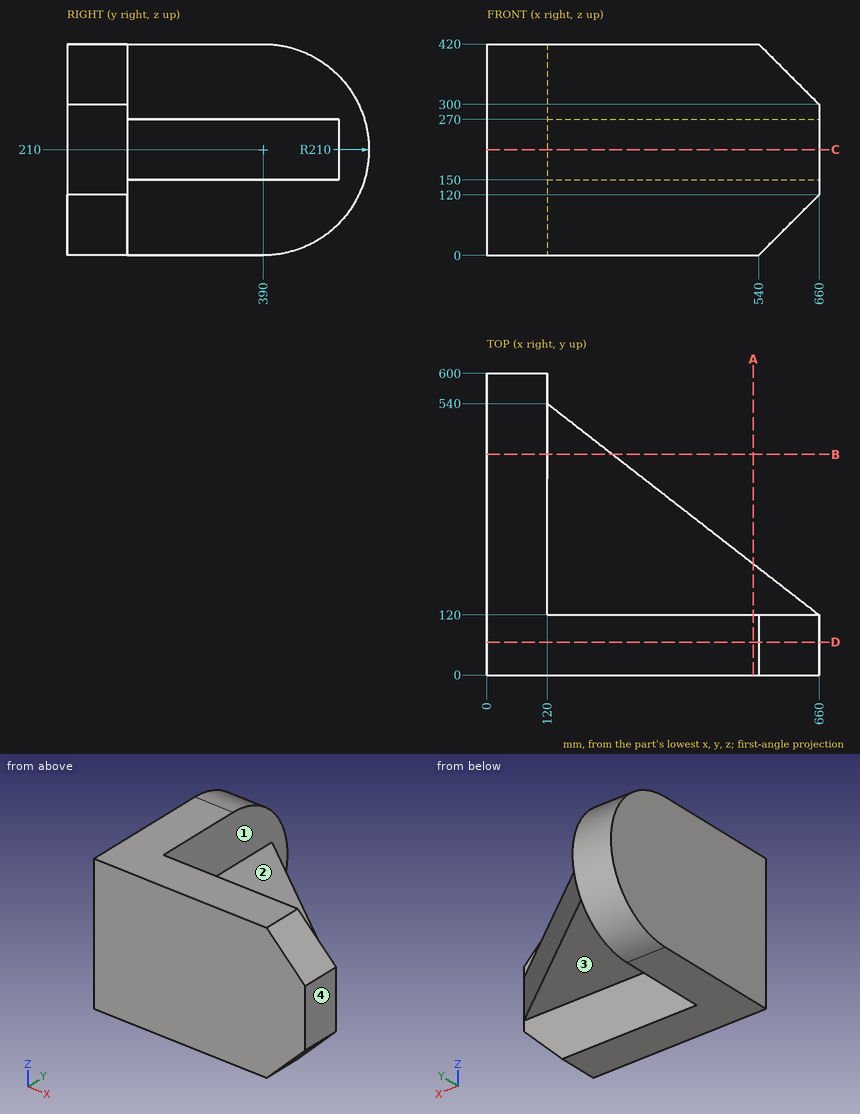
Verification items for this drawing (mm, ordinates from the low corner). A direction names the side the tool comes from. Give positions to 0.01 mm unless a question says otherwise; leave off trailing zeros. Loops run counter-clockwise (first coordinate to the right, second up) from the corner with the lowest first, then second, coordinate; pieces in that order, holes last. Notation, with made-up numbers: M 14,37.5 L 63,37.5 A24 ccw 63,61.5 Z; hole C 46.5,10.25 d2. An arc over 180 degrees is marked long. Write item = value, one per line.
(1) Sectioned sample at D-D, the plane y = 66. Record the cut outline in (x, z), plus the area to 3 significant figures.
Answer below:
outline = M 0,0 L 540,0 L 660,120 L 660,300 L 540,420 L 0,420 Z
area = 263,000 mm2
(2) Sectioned sample at B-B, the plane y = 439. Record the cut outline in (x, z).
Answer below:
outline = M 0,5.8 L 120,5.8 L 120,150 L 249.86,150 L 249.86,270 L 120,270 L 120,414.2 L 0,414.2 Z
(3) Material ranges on line 1 (Y direction, x = 154, z = 274); line 2 (Z direction, x = 182, y = 394.5), recorded low to high. Write a range as [from, to].
Answer below:
line_1 = [0, 120]
line_2 = [150, 270]
(4) Gauge pin test, flat ends, axial feed: pin 1 Ø12 at (x, y) = (183.5, 413) entering from +Z; pin 2 Ø6 at (x, y) = (226, 184) entering from -Z; pin 3 Ø5 at (y, z) = (442.5, 166.5) entering from +X. Record the tip position at first contact, or that the pin passes through.
Answer below:
pin_1 = 270
pin_2 = 150
pin_3 = 248.57
(5) Tool access check on the marked faces 1, 2, 3 and 4. Record the directions out of +Z, -Z, +X, -X, +Y, -Y that give a thin tool (end or side, any length) a straight path to the whole face; none if there is none.
Answer below:
face_1 = +X, +Y
face_2 = +Z, +X, +Y
face_3 = -Z, +X, +Y
face_4 = +Z, -Z, +X, +Y, -Y
(6) Sectioned sample at A-A, the plane x = 529.5. Record the cut outline in (y, z), plus the area to 3 significant figures.
Answer below:
outline = M 0,0 L 120,0 L 120,150 L 221.5,150 L 221.5,270 L 120,270 L 120,420 L 0,420 Z
area = 62,600 mm2
(7) Sectioned sample at C-C, the plane z = 210. Record the cut outline in (x, y).
Answer below:
outline = M 0,0 L 660,0 L 660,120 L 120,540 L 120,600 L 0,600 Z
